from build123d import *

# Parameters (mm, degrees)
SHELL1_T                 = -25.4
SHELL1_THICKNESS_2_DEPTH = 12.7
SHELL1_THICKNESS_3_DEPTH = 12.7
BOSS_EXTRUDE2_START      = -12.7
BOSS_EXTRUDE2_DEPTH      = 25.4
BOSS_EXTRUDE3_DEPTH      = 12.7


with BuildPart() as part:
    # Sketch1 → Loft1 section 0
    with BuildSketch(Plane(origin=(0, 0, 0), x_dir=(1, 0, 0), z_dir=(0, 1, 0))):
        with BuildLine():
            Line((-177.8, 165.1), (177.8, 165.1))
            Line((177.8, 165.1), (177.8, -165.1))
            Line((177.8, -165.1), (-177.8, -165.1))
            Line((-177.8, -165.1), (-177.8, 165.1))
        make_face()
    # Sketch2 → Loft1 section 1
    with BuildSketch(Plane(origin=(0, 266.7, 0), x_dir=(1, 0, 0), z_dir=(0, 1, 0))):
        with BuildLine():
            Line((-177.8, 203.2), (177.8, 203.2))
            Line((177.8, 203.2), (177.8, -203.2))
            Line((177.8, -203.2), (-177.8, -203.2))
            Line((-177.8, -203.2), (-177.8, 203.2))
        make_face()
    loft()

    # Shell1
    shell1_openings = [part.faces().sort_by_distance(p)[0] for p in [
        (0, 266.7, 0),
    ]]
    offset(amount=SHELL1_T, openings=shell1_openings, kind=Kind.INTERSECTION)

    # Shell1 thickness 2 face (on inner face of the shell) → Shell1 thickness 2 (cut)
    with BuildSketch(Plane(origin=(-152.4, 150.373987865, 0), x_dir=(0, 0, -1), z_dir=(-1, 0, 0))):
        Polygon((-143.070696797, 124.973987865), (143.070696797, 124.973987865), (177.542125368, -116.326012135), (-177.542125368, -116.326012135), align=None)
    extrude(amount=SHELL1_THICKNESS_2_DEPTH, mode=Mode.SUBTRACT)

    # Shell1 thickness 3 face (on inner face of the shell) → Shell1 thickness 3 (cut)
    with BuildSketch(Plane(origin=(152.4, 150.373987865, 0), x_dir=(0, 0, 1), z_dir=(1, 0, 0))):
        Polygon((177.542125368, -116.326012135), (-177.542125368, -116.326012135), (-143.070696797, 124.973987865), (143.070696797, 124.973987865), align=None)
    extrude(amount=SHELL1_THICKNESS_3_DEPTH, mode=Mode.SUBTRACT)

    # Sketch4 → Boss-Extrude2 (add)
    with BuildSketch(Plane(origin=(177.8, 0, 0), x_dir=(0, 0, -1), z_dir=(1, 0, 0)).offset(BOSS_EXTRUDE2_START)):
        Polygon((189.865, 266.7), (153.579285714, 12.7), (-153.579285714, 12.7), (-189.865, 266.7), align=None)
    extrude(amount=BOSS_EXTRUDE2_DEPTH)

    # Sketch5 → Boss-Extrude3 (add)
    with BuildSketch(Plane.ZY.offset(177.8)):
        Polygon((-153.579285714, 12.7), (153.579285714, 12.7), (189.865, 266.7), (-189.865, 266.7), align=None)
    extrude(amount=BOSS_EXTRUDE3_DEPTH)


solid = part.part
The model under review builds one solid part; all positions refer to its coordinate system, in mm. A direction names the side the tool comes from. Coordinates: 2 decimals unless noted, no trailing zeros. Order: outer loops, then holes, each group sorted by start corner. A loop starts at its lowest first (then second) coordinate and runs counter-clockwise, first axis right, second up. Notation, with made-up numbers: (53, 4) -> (82, 4) arc R25 cw to (82, 21) -> close; hole circle Ø3 at (86.5, 52). An arc over 180 degrees is marked (long way). Answer in a Markdown table with one row per item.
(1) Insertion check: pin 1 (12 mm diameter, centred on x = -121, z = -104.5, fed in from +Y); pin 2 (10 mm diameter, centred on x = -0.5, y = 59, fed in from -Z); pin 3 (6 mm diameter, centred on x = -9, y = 188.5, fed in from +Z). Each pin has a flat end and moves straight along its axis. Give the tip position at first contact, or say it passes through.
Answers:
| item | result |
|---|---|
| pin 1 | y = 25.4 |
| pin 2 | z = -174.24 |
| pin 3 | z = 192.46 |
(2) Consider section A-A (x = -81.5). Write out the cut boundary in (y, z), plus the area to 3 significant figures.
Answers:
| item | result |
|---|---|
| outline | (0, -165.1) -> (266.7, -203.2) -> (266.7, -177.54) -> (25.4, -143.07) -> (25.4, 143.07) -> (266.7, 177.54) -> (266.7, 203.2) -> (0, 165.1) -> close |
| area | 20,900 mm² |
(3) The part is to be moulded in two halves that separate along Z. For faces 1 (the flat face through (184, 12.7, -2)), 2 (the flat face through (0, 25.4, -4)), 3 (the flat face through (184.061, 137.922, 171.468)), say which applies: +Z half, -Z half, draft (parallel to the pull), parting line (faces both ways), or undercut.
Answers:
| item | result |
|---|---|
| face 1 | draft |
| face 2 | undercut |
| face 3 | +Z half |
(4) Machinability: for faces 4 (the flat face through (-165.1, 144, -2)), 5 (the flat face through (-184, 12.7, -2)), 6 (the flat face through (184.061, 141.478, -171.976)), 7 (the flat face through (-184.061, 137.922, 171.468)), which of the approach directions +Z, -Z, +X, -X, +Y, -Y give a long, thin tool a straight path to every point of the face, cutting with its end or side? Answer none if there is none.
Answers:
| item | result |
|---|---|
| face 4 | +Y |
| face 5 | +Z, -Z, -X, -Y |
| face 6 | -Z, +X, -Y |
| face 7 | +Z, -X, -Y |
(5) Wall thickness on line 1 along X through (y, z) = (55.5, -86.5); line 2 along Y through (x, z) = (-42, 86.5); line 3 along Z through (x, y) = (-70.5, 73): over which ranges is each line inside the solid? List them lowest first.
Answers:
| item | result |
|---|---|
| line 1 | -190.5 to -165.1, 165.1 to 190.5 |
| line 2 | 0 to 25.4 |
| line 3 | -175.53 to -149.87, 149.87 to 175.53 |
